Input: part model. Units: mm. Frame: model coordinates. Coordinates: 2 decimals unless noted, no trailing zeros. Loops run counter-clockwise (first coordinate to the right, second up) from the corner with the lowest first, then second, coordinate; pieces in that order, holes last. Notation, with made-up numbers: (71, -39) - (77, -39) arc R29 ccw to (77, -17) - close; hole circle Ø10 at (41, -31). An arc over 180 degrees is marked (long way). Use one line per item in the form item = value.
Autodesk Inventor part; units mm, degrees
ref_plane "YZ Plane" through (0, 0, 0) normal (1, 0, 0) x (0, 1, 0)
ref_plane "XZ Plane" through (0, 0, 0) normal (0, 1, 0) x (-1, 0, 0)
ref_plane "XY Plane" through (0, 0, 0) normal (0, 0, 1) x (1, 0, 0)
sketch "Sketch1" plane through (0, 0, 0) normal (0, 0, 1) x (1, 0, 0)
  line L0 (0, 0) -> (50, 0)
  line L1 (0, 0) -> (-91.9239, 91.9239)
  line L2 (0, 0) -> (130, 0) construction
  line L3 (-91.9239, 91.9239) -> (-90.1561, 93.6916)
  line L4 (-91.9239, 91.9239) -> (-89.4239, 91.9239) construction
  line L5 (-90.1561, 93.6916) -> (1.0355, 2.5)
  line L6 (50, 0) -> (50, 2.5)
  line L7 (50, 2.5) -> (1.0355, 2.5)
  dimension "d0" = 50
  dimension "d1" = 130
  dimension "d2" = 135
  dimension "d3" = 2.5
  dimension "d4" = 45
  dimension "d5" = 90
  dimension "d6" = 2.5
extrude "Extrusion1" add sketch "Sketch1" along normal blind 10
sketch "Sketch2" plane through (0, 0, 0) normal (0, -1, 0) x (1, 0, 0)
  line L0 (0, 0) -> (0, 10)
  line L1 (0, 5) -> (30, 5)
  circle A0 centre (30, 5) radius 2
  dimension "d9" = 30
  dimension "d10" = 4
extrude "Extrusion2" cut sketch "Sketch2" against normal blind 10
sketch "Sketch3" plane through (0, 0, 10) normal (-0.7071, -0.7071, 0) x (-0.7071, 0.7071, 0)
  line L0 (0, 10) -> (0, 0)
  line L1 (0, 5) -> (50, 5)
  line L2 (0, 5) -> (50, 5) construction
  line L3 (50, 5) -> (100, 5)
  line L4 (50, 5) -> (100, 5) construction
  circle A0 centre (100, 5) radius 2
  circle A1 centre (50, 5) radius 2
  dimension "d13" = 50
  dimension "d14" = 0
  dimension "d15" = 50
  dimension "d16" = 0
  dimension "d17" = 4
  dimension "d18" = 4
extrude "Extrusion3" cut sketch "Sketch3" against normal blind 10
properties part number "ChassisClamp"
Q1. Cut plane D-D, the plane y = 17.5. Return loops of the section in (x, z), then the cut area to 3 significant figures.
Check values:
outline = (-17.5, 0) - (-13.96, 0) - (-13.96, 10) - (-17.5, 10) - close
area = 35.4 mm²
Q2. Cut plane C-C, the plane x = 11. Return loops of the section in (y, z).
Check values:
outline = (0, 0) - (2.5, 0) - (2.5, 10) - (0, 10) - close
Q3. Cut plane A-A, the plane x = 30. Return loops of the section in (y, z), then the cut area to 3 significant figures.
Check values:
outline = (0, 0) - (2.5, 0) - (2.5, 3) - (0, 3) - close; (0, 7) - (2.5, 7) - (2.5, 10) - (0, 10) - close
area = 15.0 mm²
Q4. First-contact query: P1, Ø2, axis at x = -66.5, z = 4, coming from the -Y side; P2, Ø2, axis at x = 34, z = 4.5, coming from the -Y side; P3, Ø1.5, axis at y = 27.5, z = 5.5, coming from the -X side; P4, Ø2, axis at y = 61.5, z = 5, coming from the +X side. Flat tips, straight axial feed; report the tip coordinate or a pass-through.
Check values:
P1 = 65.5
P2 = 0
P3 = -28.25
P4 = -56.96
Q5. Cut plane B-B, the plane z = 5. Return loops of the section in (x, y), then the cut area to 3 significant figures.
Check values:
outline = (-91.92, 91.92) - (-72.12, 72.12) - (-70.36, 73.89) - (-90.16, 93.69) - close; (-69.3, 69.3) - (-36.77, 36.77) - (-35, 38.54) - (-67.53, 71.06) - close; (-33.94, 33.94) - (0, 0) - (28, 0) - (28, 2.5) - (1.04, 2.5) - (-32.17, 35.71) - close; (32, 0) - (50, 0) - (50, 2.5) - (32, 2.5) - close
area = 417 mm²
Q6. Ray query, line 1 along Z through (x, y) = (30, 1); line 2 along Y through (x, z) = (13.5, 5.75); line 3 along X through (y, z) = (0.9, 5). Return the intervals inside material, ascending. Write a range as [from, to].
Check values:
line_1 = [0, 3], [7, 10]
line_2 = [0, 2.5]
line_3 = [-0.9, 28], [32, 50]
Q7. Pull-direction query (Y, two-part tool) for faces 1 (the cylindrical face through (31.908, 1.232, 5.601)), 2 (the cylindrical face through (-68.426, 70.169, 4.912)), 3 (the flat face through (25, 0, 5)), 4 (the flat face through (26, 2.5, 5)); classes: pulls with the +Y half, pulls with the -Y half, needs draft (parallel to the pull), parting line crosses it, or undercut.
Check values:
face_1 = needs draft
face_2 = undercut
face_3 = pulls with the -Y half
face_4 = pulls with the +Y half
